from build123d import *

# Parameters (mm, degrees)
BOSS_EXTRUDE1_DEPTH      = 12
BOSS_EXTRUDE1_DEPTH_BACK = 12
SKETCH1_R                = 7.5
CUT_EXTRUDE1_DEPTH       = 183.477874792
CUT_EXTRUDE1_DEPTH_BACK  = 183.477874792
SKETCH2_W                = 16
SKETCH2_H                = 95.07


with BuildPart() as part:
    # Sketch1 → Boss-Extrude1 (new, two sides: drawn at the far end of the back side and taken through both)
    with BuildSketch(Plane.XY.offset(-BOSS_EXTRUDE1_DEPTH_BACK)):
        with BuildLine():
            ThreePointArc((-49.084636864, 6.747346105), (-67.717886444, -3.252653895), (-49.084636864, -13.252653895))
            Line((-49.084636864, -13.252653895), (137.648863975, -13.252653895))
            ThreePointArc((137.648863975, -13.252653895), (156.282113556, -3.252653895), (137.648863975, 6.747346105))
            Line((137.648863975, 6.747346105), (23.712113556, 6.747346105))
            Line((23.712113556, 6.747346105), (23.712113556, 109.817346105))
            Line((23.712113556, 109.817346105), (46.212113556, 109.817346105))
            Line((46.212113556, 109.817346105), (46.212113556, 124.817346105))
            Line((46.212113556, 124.817346105), (-18.787886444, 124.817346105))
            Line((-18.787886444, 124.817346105), (-18.787886444, 109.817346105))
            Line((-18.787886444, 109.817346105), (3.712113556, 109.817346105))
            Line((3.712113556, 109.817346105), (3.712113556, 6.747346105))
            Line((3.712113556, 6.747346105), (-49.084636864, 6.747346105))
        make_face()
        with Locations((-55.717886444, -3.252653895)):
            Circle(SKETCH1_R, mode=Mode.SUBTRACT)
        with Locations((144.282113556, -3.252653895)):
            Circle(SKETCH1_R, mode=Mode.SUBTRACT)
    extrude(amount=BOSS_EXTRUDE1_DEPTH + BOSS_EXTRUDE1_DEPTH_BACK)

    # Sketch2 → Cut-Extrude1 (cut, two sides: drawn at the far end of the back side and taken through both)
    with BuildSketch(Plane(origin=(23.712113556, 0, 0), x_dir=(0, 0, -1), z_dir=(1, 0, 0)).offset(-CUT_EXTRUDE1_DEPTH_BACK)):
        with Locations((0, 58.282346105)):
            Rectangle(SKETCH2_W, SKETCH2_H)
    extrude(amount=CUT_EXTRUDE1_DEPTH + CUT_EXTRUDE1_DEPTH_BACK, mode=Mode.SUBTRACT)


solid = part.part
Geometry check sheet. Reference: the model listing, model coordinates, mm. A direction names the side the tool comes from. Coordinates: 2 decimals unless noted, no trailing zeros. Order: outer loops, then holes, each group sorted by start corner. A loop starts at its lowest first (then second) coordinate and runs counter-clockwise, first axis right, second up. Notation, with made-up numbers: (14, -23.5) - (59, -23.5) arc R37 ccw to (59, 13.5) - close; hole circle Ø9 at (68.5, 63.25). An arc over 180 degrees is marked (long way). One line per item, written item: value.
(1) Sectioned sample at B-B (y = 53.5). Enter the section's corners in (x, z).
Data:
outline: (3.71, -12) - (23.71, -12) - (23.71, -8) - (3.71, -8) - close; (3.71, 8) - (23.71, 8) - (23.71, 12) - (3.71, 12) - close
(2) Access from +Z, -Z, +X, -X, +Y, -Y to the whole of each face (thin tool, end or side, straight path). Record for faces 1 (the face through (81, 6.747, 0)), 2 (the face through (14, 10.747, 0)), 3 (the face through (43, -13.253, 0)), 4 (the face through (-8, 109.817, 0)), 5 (the face through (19, 29, -12)).
Data:
face 1: +Z, -Z
face 2: +X, -X
face 3: +Z, -Z, -Y
face 4: +Z, -Z, -X
face 5: -Z, +X, -X, +Y, -Y
(3) Thickness scan on probe 1 along X at (y, z) = (-1, -9.25); probe 2 along Z at (x, y) = (20, 83); probe 3 along Y at (x, z) = (6.5, -3.5). Record the ranges inside material, lowest first. Write a range as from..to.
Data:
probe 1: x = -67.5..-62.87, -48.56..137.13, 151.44..156.07
probe 2: z = -12..-8, 8..12
probe 3: y = -13.25..10.75, 105.82..124.82
(4) Sectioned sample at C-C (z = -2.5). Enter the section's corners in (x, y).
Data:
outline: (-49.08, -13.25) - (137.65, -13.25) arc R12 ccw (long way) to (137.65, 6.75) - (23.71, 6.75) - (23.71, 10.75) - (3.71, 10.75) - (3.71, 6.75) - (-49.08, 6.75) arc R12 ccw (long way) to start; (-18.79, 109.82) - (3.71, 109.82) - (3.71, 105.82) - (23.71, 105.82) - (23.71, 109.82) - (46.21, 109.82) - (46.21, 124.82) - (-18.79, 124.82) - close; hole circle Ø15 at (-55.72, -3.25); hole circle Ø15 at (144.28, -3.25)
(5) Sectioned sample at A-A (x = -11). Enter the section's corners in (y, z).
Data:
outline: (-13.25, -12) - (6.75, -12) - (6.75, 12) - (-13.25, 12) - close; (109.82, -12) - (124.82, -12) - (124.82, 12) - (109.82, 12) - close
(6) Release check for a two-part mould opening along X. For faces 6 (the face through (14, 58, -8)), 7 (the face through (46.212, 117, 0)), 8 (the face through (-18.788, 117, 0)), 9 (the face through (156.277, -3.615, -0.168)) record: +X half, -X half, draft (parallel to the pull), parting line (faces both ways), or undercut.
Data:
face 6: draft
face 7: +X half
face 8: -X half
face 9: undercut
(7) Sectioned sample at D-D (y = 2). Enter the section's corners in (x, z), and give its area (3 significant figures).
Data:
outline: (-66.51, -12) - (-61.07, -12) - (-61.07, 12) - (-66.51, 12) - close; (-50.36, -12) - (138.93, -12) - (138.93, 12) - (-50.36, 12) - close; (149.64, -12) - (155.07, -12) - (155.07, 12) - (149.64, 12) - close
area: 4,800 mm^2
(8) Depth check by flat-ended pin: pin 1 Ø10 at (x, z) = (-5, 2.5) entering from -Y; pin 2 Ø9 at (x, y) = (-55.72, -3.25) entering from -Z; pin 3 Ø4.5 at (y, z) = (117.5, -5.5) entering from +X; pin 4 Ø6 at (y, z) = (2.5, -6.5) entering from +X. Enter the tip coordinate at first touch or a pass-through.
Data:
pin 1: stops at y = -13.25
pin 2: passes through
pin 3: stops at x = 46.21
pin 4: stops at x = 155.96
